from build123d import *

# Parameters (mm, degrees)
F0_W     = 12.7
F0_H     = 8.763
F1_DEPTH = 3.175
F3_DEPTH = 8.763
F4_R     = 1.8415
F5_DEPTH = 25.4
F6_R     = 3.683
F6_R_2   = 1.8415
F7_DEPTH = 2.286
F8_W     = 12.7
F8_H     = 8.763
F8_R     = 1.8415
F9_DEPTH = 1.524


with BuildPart() as f1:
    # F0 (on Top) → F1 (new body)
    with BuildSketch(Plane.XY):
        Rectangle(F0_W, F0_H)
    extrude(amount=F1_DEPTH)

    # F2 (on face) → F3 (join)
    with BuildSketch(Plane.XZ.offset(4.3815)):
        Polygon((-6.35, 3.175), (6.35, 3.175), (6.35, 6.35), (-11.43, 6.35), (-11.43, 3.175), align=None)
    extrude(amount=-F3_DEPTH)

    # F4 (on face) → F5 (cut)
    with BuildSketch(Plane.XY.offset(6.35)):
        Circle(F4_R)
    extrude(amount=-F5_DEPTH, mode=Mode.SUBTRACT)

    # F6 (on face) → F7 (cut)
    with BuildSketch(Plane.XY.offset(6.35)):
        Circle(F6_R)
        Circle(F6_R_2, mode=Mode.SUBTRACT)
    extrude(amount=-F7_DEPTH, mode=Mode.SUBTRACT)

    # F8 (on face) → F9 (join)
    with BuildSketch(Plane(origin=(0, 0, 0), x_dir=(1, 0, 0), z_dir=(0, 0, -1))):
        Rectangle(F8_W, F8_H)
        Circle(F8_R, mode=Mode.SUBTRACT)
    extrude(amount=F9_DEPTH)


solid = f1.part
Could you check a few things on this model? Use its own coordinates, in mm. A direction names the side the tool comes from. Round coordinates to 2 decimals unless told otherwise and drop trailing zeros. Write each loop counter-clockwise with the first axis right and the second up, starting at its lowest first coordinate (ties: lowest second). Pieces come first, ordered by that corner, then holes. Notation, with made-up numbers: (-18.75, 36) - (14.25, 36) arc R36 cw to (14.25, 70) - close; hole circle Ø4 at (14, 80.5). An arc over 180 degrees is marked (long way). Put each result on its own line as item: value. Start each with the question number.
(1) Will these pins go through, and if not, where does the flat tip stop? pin 1 (2 mm diameter, centred on y = 0, z = 0, fed in from -X); pin 2 (3.5 mm diameter, centred on x = -0.5, y = 1, fed in from +Z); pin 3 (3 mm diameter, centred on x = -9, z = 0, fed in from -Y).
(2) I want a section at D-D, the plane x = 3. Please give me the cut outline in (y, z), plus the area to 3 significant figures.
(3) I need wall thicknesses on probe 1 along Y at (x, z) = (0, 2.5); probe 2 along X at (y, z) = (0, 0.25); probe 3 along Z at (x, y) = (-2, 1.5). Which ranges of each line are inside material? Lowest first, please.
(4) I want a section at C-C, the plane z = -0.5. Please give me the cut outline in (x, y).
(5) For faces 5 (the flat face through (-9, 0, 3.175)), 6 (the flat face through (-4, 0, 6.35)), 7 (the cylindrical face through (1.699, -3.267, 5.223)), which set-ups out of +Z, -Z, +X, -X, +Y, -Y let a thin tool reach every point of the face, with its end or its side?
(6) I want a section at B-B, the plane x = 0. Please give me the cut outline in (y, z), plus the area to 3 significant figures.
(7) Thinking about a two-plate mould opening in Y: for faces 1 (the flat face through (-6.35, 0, 1)), 2 (the flat face through (-1, -4.382, 2)), 3 (the flat face through (1, 2, 4.064)), 4 (the flat face through (-1, 4.382, 2)), which applies, released by +Y, released by -Y, zero draft, split by the parting line, or undercut?
Here are the results:
1. pin 1: stops at x = -6.35
1. pin 2: stops at z = 4.06
1. pin 3: passes through
2. outline: (-4.38, -1.52) - (4.38, -1.52) - (4.38, 6.35) - (2.14, 6.35) - (2.14, 4.06) - (-2.14, 4.06) - (-2.14, 6.35) - (-4.38, 6.35) - close
2. area: 59.2 mm^2
3. probe 1: y = -4.38 to -1.84, 1.84 to 4.38
3. probe 2: x = -6.35 to -1.84, 1.84 to 6.35
3. probe 3: z = -1.52 to 4.06
4. outline: (-6.35, -4.38) - (6.35, -4.38) - (6.35, 4.38) - (-6.35, 4.38) - close; hole circle Ø3.68 at (0, 0)
5. face 5: -Z, -X, +Y, -Y
5. face 6: +Z, +X, -X, +Y, -Y
5. face 7: +Z
6. outline: (-4.38, -1.52) - (-1.84, -1.52) - (-1.84, 4.06) - (-3.68, 4.06) - (-3.68, 6.35) - (-4.38, 6.35) - close; (1.84, -1.52) - (4.38, -1.52) - (4.38, 6.35) - (3.68, 6.35) - (3.68, 4.06) - (1.84, 4.06) - close
6. area: 31.6 mm^2
7. face 1: zero draft
7. face 2: released by -Y
7. face 3: undercut
7. face 4: released by +Y
